For this review, take the finished solid that the model builds, in its own axes (mm). A direction names the side the tool comes from. Coordinates: 2 decimals unless noted, no trailing zeros. Order: outer loops, then holes, each group sorted by start corner. A loop starts at its lowest first (then second) coordinate and runs counter-clockwise, first axis right, second up. Notation, with made-up numbers: (-1.5, -15.5) -> (55.5, -15.5) arc R20 ccw to (55.5, -4.5) -> close; hole circle Ø9 at (39.5, 23). An arc over 180 degrees is marked (long way). Write item = value, one per line. Start each with the question number.
1) Draft analysis for pull direction X (two halves, no side actions). For faces 1 (the face through (-44.5, 9, 19.4)), 2 (the face through (-46, 4, -31)), 3 (the face through (-37, 1, -18.75)), state which applies: +X half, -X half, draft (parallel to the pull), parting line (faces both ways), or undercut.
2) Machinability: for faces 4 (the face through (6, 1, -6)), 5 (the face through (-19, 1, -31)), 6 (the face through (-37, 1, 17.25)), which of the approach directions +Z, -Z, +X, -X, +Y, -Y give a long, thin tool a straight path to every point of the face, cutting with its end or side? Answer none if there is none.
3) Consider section B-B on y = 3.25. Give the boundary of the cut face in (x, z), and give its area (3 significant figures).
4) Insertion check: pin 1 Ø1.6 at (x, y) = (-11.5, 0.5) entering from -Z; pin 2 Ø2 at (x, y) = (-22, 1.5) entering from +Z; pin 3 Ø1 at (y, z) = (1, -11.5) entering from +X; pin 4 Ø3 at (y, z) = (4.5, -2.5) entering from +X. Each pin has a flat end and moves straight along its axis. Give the tip position at first contact, or say it passes through.
5) Consider section A-A on x = -9.5. Give the boundary of the cut face in (y, z).
6) Wall thickness on probe 1 along X at (y, z) = (1, -21.5); probe 2 along Y at (x, z) = (-2.5, 18): over which ranges is each line inside the solid? List them lowest first. Write a range as [from, to].
7) Consider section D-D on x = -31. Give the boundary of the cut face in (y, z), and give its area (3 significant figures).
8) Consider section C-C on z = -11. Give the boundary of the cut face in (x, y), and give its area (3 significant figures).
from build123d import *

# Parameters (mm, degrees)
SKETCH1_W           = 50
SKETCH1_H           = 50
SKETCH1_W_2         = 10.5
SKETCH1_H_2         = 10.5
BOSS_EXTRUDE1_DEPTH = 2
BOSS_EXTRUDE2_DEPTH = 9


with BuildPart() as part:
    # Sketch1 → Boss-Extrude1 (new body)
    with BuildSketch(Plane(origin=(0, 0, 0), x_dir=(1, 0, 0), z_dir=(0, 1, 0))):
        with Locations((-19, 6)):
            Rectangle(SKETCH1_W, SKETCH1_H)
        with Locations((-25, 24)):
            Rectangle(SKETCH1_W_2, SKETCH1_H_2, mode=Mode.SUBTRACT)
        with Locations((-37, 12)):
            Rectangle(SKETCH1_W_2, SKETCH1_H_2, mode=Mode.SUBTRACT)
        with Locations((-37, 24)):
            Rectangle(SKETCH1_W_2, SKETCH1_H_2, mode=Mode.SUBTRACT)
        with Locations((-13, 24)):
            Rectangle(SKETCH1_W_2, SKETCH1_H_2, mode=Mode.SUBTRACT)
        with Locations((-1, 24)):
            Rectangle(SKETCH1_W_2, SKETCH1_H_2, mode=Mode.SUBTRACT)
        with Locations((-37, 0)):
            Rectangle(SKETCH1_W_2, SKETCH1_H_2, mode=Mode.SUBTRACT)
        with Locations((-37, -12)):
            Rectangle(SKETCH1_W_2, SKETCH1_H_2, mode=Mode.SUBTRACT)
        with Locations((-25, 12)):
            Rectangle(SKETCH1_W_2, SKETCH1_H_2, mode=Mode.SUBTRACT)
        with Locations((-25, 0)):
            Rectangle(SKETCH1_W_2, SKETCH1_H_2, mode=Mode.SUBTRACT)
        with Locations((-13, 12)):
            Rectangle(SKETCH1_W_2, SKETCH1_H_2, mode=Mode.SUBTRACT)
        with Locations((-1, 12)):
            Rectangle(SKETCH1_W_2, SKETCH1_H_2, mode=Mode.SUBTRACT)
        with Locations((-13, 0)):
            Rectangle(SKETCH1_W_2, SKETCH1_H_2, mode=Mode.SUBTRACT)
        with Locations((-1, 0)):
            Rectangle(SKETCH1_W_2, SKETCH1_H_2, mode=Mode.SUBTRACT)
        with Locations((-25, -12)):
            Rectangle(SKETCH1_W_2, SKETCH1_H_2, mode=Mode.SUBTRACT)
        with Locations((-13, -12)):
            Rectangle(SKETCH1_W_2, SKETCH1_H_2, mode=Mode.SUBTRACT)
        with Locations((-1, -12)):
            Rectangle(SKETCH1_W_2, SKETCH1_H_2, mode=Mode.SUBTRACT)
    extrude(amount=BOSS_EXTRUDE1_DEPTH)

    # Sketch1_32 → Boss-Extrude2 (add)
    with BuildSketch(Plane(origin=(0, 0, 0), x_dir=(1, 0, 0), z_dir=(0, 1, 0))):
        Polygon((4, 33), (4, 31), (6, 31), (6, 29), (8, 29), (8, 33), align=None)
        Polygon((-44, 31), (-42, 31), (-42, 33), (-46, 33), (-46, 29), (-44, 29), align=None)
        Polygon((-44, -19), (-44, -17), (-46, -17), (-46, -21), (-42, -21), (-42, -19), align=None)
        Polygon((8, -17), (6, -17), (6, -19), (4, -19), (4, -21), (8, -21), align=None)
    extrude(amount=BOSS_EXTRUDE2_DEPTH)


solid = part.part
Answer sheet:
q1.face_1 = draft
q1.face_2 = -X half
q1.face_3 = undercut
q2.face_4 = +X, +Y, -Y
q2.face_5 = -Z, +Y, -Y
q2.face_6 = +Y, -Y
q3.outline = (-46, -33) -> (-42, -33) -> (-42, -31) -> (-44, -31) -> (-44, -29) -> (-46, -29) -> close; (-46, 17) -> (-44, 17) -> (-44, 19) -> (-42, 19) -> (-42, 21) -> (-46, 21) -> close; (4, -33) -> (8, -33) -> (8, -29) -> (6, -29) -> (6, -31) -> (4, -31) -> close; (4, 19) -> (6, 19) -> (6, 17) -> (8, 17) -> (8, 21) -> (4, 21) -> close
q3.area = 48.0 mm2
q4.pin_1 = -31
q4.pin_2 = 19
q4.pin_3 = 6
q4.pin_4 = through
q5.outline = (0, -31) -> (2, -31) -> (2, -29.25) -> (0, -29.25) -> close; (0, -18.75) -> (2, -18.75) -> (2, -17.25) -> (0, -17.25) -> close; (0, -6.75) -> (2, -6.75) -> (2, -5.25) -> (0, -5.25) -> close; (0, 5.25) -> (2, 5.25) -> (2, 6.75) -> (0, 6.75) -> close; (0, 17.25) -> (2, 17.25) -> (2, 19) -> (0, 19) -> close
q6.probe_1 = [-44, -42.25], [-31.75, -30.25], [-19.75, -18.25], [-7.75, -6.25], [4.25, 6]
q6.probe_2 = [0, 2]
q7.outline = (0, -31) -> (2, -31) -> (2, 19) -> (0, 19) -> close
q7.area = 100 mm2
q8.outline = (-44, 0) -> (-42.25, 0) -> (-42.25, 2) -> (-44, 2) -> close; (-31.75, 0) -> (-30.25, 0) -> (-30.25, 2) -> (-31.75, 2) -> close; (-19.75, 0) -> (-18.25, 0) -> (-18.25, 2) -> (-19.75, 2) -> close; (-7.75, 0) -> (-6.25, 0) -> (-6.25, 2) -> (-7.75, 2) -> close; (4.25, 0) -> (6, 0) -> (6, 2) -> (4.25, 2) -> close
q8.area = 16.0 mm2
